Geometry: final body of the model. Coordinates: model frame, mm. Face numbers are marked on the shaded views. Round coordinates to 2 decimals unless told otherwise and drop trailing zeros. Write each loop counter-clockwise with the first axis right and the second up, starting at its lowest first coordinate (ties: lowest second). Pieces come first, ordered by that corner, then holes. Notation, with made-up numbers: (57, 28.25) -> (88, 28.25) arc R20 cw to (88, 32.25) -> close; hole circle Ø3 at (50, -30). An arc over 180 degrees is marked (long way). Use one line per item in the form item = value. Start each with the question number.
1. Line query: L1, parallel to X at y = -2.25, z = 5; L2, parallel to X at y = -5.5, z = -13.5; L3, parallel to Z at x = 61, y = -1.25. Output: solid intervals per line, ascending.
2. Cut plane C-C, the plane y = -8.5. State how many separate pieces and enclosed holes the cut face has, plus the area to 3 significant figures.
3. Cut plane D-D, the plane z = 43.5. Return the cut outline in (x, y).
4. Pin query (flat end, axial travel): pin 1 Ø12 at (x, z) = (-26, 16) entering from -Y; pin 2 Ø3 at (y, z) = (-8.5, -22) entering from +X; pin 3 Ø1 at (x, y) = (40.5, -7) entering from +Z; pin 4 Ø1 at (y, z) = (-6, 14) entering from +X. Return the tip coordinate at first contact, or that it passes through.
5. Cut plane A-A, the plane x = -35. Return the cut outline in (y, z), plus the area to 3 significant figures.
6. Cut plane B-B, the plane z = 0. Return the cut outline in (x, y), plus the area to 3 significant figures.
7. Draft query along Z for the marked faces 1, 2 and 3. Return one class per face: pulls with the +Z half, pulls with the -Z half, needs draft (parallel to the pull), parting line crosses it, or undercut.
```python
from build123d import *

# Parameters (mm, degrees)
F0_R     = 3.4
F0_R_2   = 28.2
F1_DEPTH = 10


with BuildPart() as f1:
    # F0 (on Front) → F1 (new body)
    with BuildSketch(Plane.XZ):
        with BuildLine():
            ThreePointArc((65, -40), (72.936036, 32.570802), (0, 35.707142))
            ThreePointArc((0, 35.707142), (-72.936036, 32.570802), (-65, -40))
            Line((-65, -40), (65, -40))
        make_face()
        with Locations((-63.284271, -28.284271)):
            Circle(F0_R, mode=Mode.SUBTRACT)
        with Locations((-6.715729, -28.284271)):
            Circle(F0_R, mode=Mode.SUBTRACT)
        with Locations((-35, 0)):
            Circle(F0_R_2, mode=Mode.SUBTRACT)
        with Locations((6.819313, -28.387856)):
            Circle(F0_R, mode=Mode.SUBTRACT)
        with Locations((63.49144, -28.284271)):
            Circle(F0_R, mode=Mode.SUBTRACT)
        with Locations((35.103584, 0)):
            Circle(F0_R_2, mode=Mode.SUBTRACT)
        with Locations((-63.284271, 28.284271)):
            Circle(F0_R, mode=Mode.SUBTRACT)
        with Locations((-6.715729, 28.284271)):
            Circle(F0_R, mode=Mode.SUBTRACT)
        with Locations((6.715729, 28.284271)):
            Circle(F0_R, mode=Mode.SUBTRACT)
        with Locations((63.387856, 28.387856)):
            Circle(F0_R, mode=Mode.SUBTRACT)
    extrude(amount=F1_DEPTH)


solid = f1.part
```
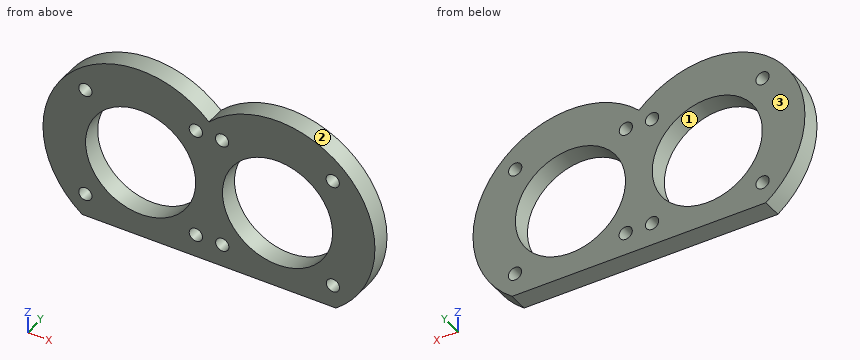
Outcome:
q1.L1 = -84.75 to -62.75, -7.25 to 7.35, 62.86 to 84.75
q1.L2 = -83.14 to -59.76, -10.24 to 10.34, 59.86 to 83.14
q1.L3 = -40 to -30.6, -25.97 to -11.16, 11.16 to 25.97, 30.81 to 42.71
q2.separate_pieces = 1
q2.enclosed_holes = 10
q2.area = 8,150 mm^2
q3.outline = (-59.65, -10) -> (-10.35, -10) -> (-10.35, 0) -> (-59.65, 0) -> close; (10.35, -10) -> (59.65, -10) -> (59.65, 0) -> (10.35, 0) -> close
q4.pin_1 = through
q4.pin_2 = 80.6
q4.pin_3 = 49.75
q4.pin_4 = 83.14
q5.outline = (-10, -40) -> (0, -40) -> (0, -28.2) -> (-10, -28.2) -> close; (-10, 28.2) -> (0, 28.2) -> (0, 50) -> (-10, 50) -> close
q5.area = 336 mm^2
q6.outline = (-85, -10) -> (-63.2, -10) -> (-63.2, 0) -> (-85, 0) -> close; (-6.8, -10) -> (6.9, -10) -> (6.9, 0) -> (-6.8, 0) -> close; (63.3, -10) -> (85, -10) -> (85, 0) -> (63.3, 0) -> close
q6.area = 572 mm^2
q7.face_1 = undercut
q7.face_2 = parting line crosses it
q7.face_3 = needs draft
